Autodesk Inventor part; units mm, degrees
ref_plane "YZ Plane" through (0, 0, 0) normal (1, 0, 0) x (0, 1, 0)
ref_plane "XZ Plane" through (0, 0, 0) normal (0, 1, 0) x (-1, 0, 0)
ref_plane "XY Plane" through (0, 0, 0) normal (0, 0, 1) x (1, 0, 0)
sketch "Sketch1" plane through (0, 0, 0) normal (0, 1, 0) x (-1, 0, 0)
  circle A0 centre (0, 0) radius 12.7
  dimension "d0" = 25.4
extrude "Extrusion1" add sketch "Sketch1" along normal blind 25.4
sketch "Sketch2" plane through (0, 25.4, 0) normal (0, 1, 0) x (1, 0, 0)
  circle A0 centre (0, 0) radius 15.875
  dimension "d3" = 31.75
extrude "Extrusion2" add sketch "Sketch2" along normal blind 5.08
sketch "Sketch3" plane through (0, 0, 0) normal (0, -1, 0) x (1, 0, 0)
  circle A0 centre (0, 0) radius 12.7
extrude "Extrusion3" add sketch "Sketch3" along normal blind 6.35
chamfer "Chamfer1" distance 3.175 distance2 6.35 1 edges at (-12.7, -6.35, 0) measured on face at (0.3934, -6.35, -3.2397)
sketch "Sketch4" plane through (0, 30.48, 0) normal (0, 1, 0) x (1, 0, 0)
  line L0 (0, 0) -> (1.016, 0) construction
  line L1 (0, 0) -> (-1.016, 0) construction
  line L2 (-1.016, 0) -> (-3.556, 0) construction
  line L3 (-3.556, 0) -> (-3.556, 6.35) construction
  line L4 (-3.556, 6.35) -> (-1.016, 6.35) construction
  line L5 (-1.016, 6.35) -> (-1.016, 0) construction
  line L6 (-1.016, 6.35) -> (-6.096, 6.35)
  line L7 (-6.096, 6.35) -> (-6.096, -6.35)
  line L8 (-6.096, -6.35) -> (-1.016, -6.35)
  line L9 (-1.016, -6.35) -> (-1.016, 6.35)
  line L10 (1.016, 0) -> (1.016, 7.239) construction
  line L11 (1.016, 0) -> (6.096, 0) construction
  line L12 (3.556, 0) -> (3.556, 4.572) construction
  line L13 (3.556, 0) -> (3.556, -4.572) construction
  line L14 (3.556, 4.572) -> (4.826, 4.572) construction
  line L15 (3.556, -4.572) -> (2.286, -4.572) construction
  line L16 (4.826, 4.572) -> (3.556, 4.572)
  line L17 (3.556, 4.572) -> (3.556, -4.572)
  line L18 (3.556, -4.572) -> (4.826, -4.572)
  line L19 (4.826, -4.572) -> (4.826, 4.572)
  line L20 (1.016, 7.239) -> (6.096, 7.239) construction
  line L21 (6.096, 7.239) -> (3.5838, 7.239)
  line L22 (1.016, 4.6712) -> (1.016, -4.6712)
  line L23 (3.5838, -7.239) -> (6.096, -7.239)
  line L24 (6.096, -7.239) -> (6.096, 7.239)
  line L25 (-2.286, 0) -> (-3.556, 0)
  line L26 (-3.556, 0) -> (-3.556, 5.08)
  line L27 (-3.556, 5.08) -> (-2.286, 5.08)
  line L28 (-2.286, 5.08) -> (-2.286, 0)
  line L29 (-2.286, 0) -> (-3.556, 0)
  line L30 (-3.556, 0) -> (-3.556, -5.08)
  line L31 (-3.556, -5.08) -> (-2.286, -5.08)
  line L32 (-2.286, -5.08) -> (-2.286, 0)
  line L33 (1.016, 7.239) -> (1.016, 5.334) construction
  line L34 (1.016, -7.239) -> (1.016, -5.334) construction
  line L35 (1.016, -7.239) -> (2.921, -7.239) construction
  line L36 (1.016, 7.239) -> (2.921, 7.239) construction
  line L37 (2.4523, 6.7703) -> (1.4847, 5.8027)
  line L38 (1.4847, -5.8027) -> (2.4523, -6.7703)
  arc A0 (3.5838, 7.239) -> (2.4523, 6.7703) centre (3.5838, 5.6388) ccw
  arc A1 (1.4847, 5.8027) -> (1.016, 4.6712) centre (2.6162, 4.6712) ccw
  arc A2 (1.016, -4.6712) -> (1.4847, -5.8027) centre (2.6162, -4.6712) ccw
  arc A3 (2.4523, -6.7703) -> (3.5838, -7.239) centre (3.5838, -5.6388) ccw
  dimension "d11" = 1.016
  dimension "d12" = 1.016
  dimension "d13" = 2.54
  dimension "d14" = 6.35
  dimension "d15" = 5.08
  dimension "d16" = 12.7
  dimension "d17" = 7.239
  dimension "d18" = 5.08
  dimension "d19" = 4.572
  dimension "d20" = 4.572
  dimension "d21" = 1.27
  dimension "d22" = 1.27
  dimension "d23" = 5.08
  dimension "d24" = 14.478
  dimension "d25" = 5.08
  dimension "d26" = 5.08
  dimension "d27" = 1.905
  dimension "d28" = 1.905
  dimension "d29" = 1.905
  dimension "d30" = 1.905
  dimension "d31" = 1.6002
extrude "Extrusion4" cut sketch "Sketch4" against normal blind 6.35
properties part number "usbHdmiPanelMount" material "ABS Plastic"
The model under review builds one solid part; all positions refer to its coordinate system, in mm. A direction names the side the tool comes from. Round coordinates to 2 decimals unless told otherwise and drop trailing zeros. Loops run counter-clockwise (first coordinate to the right, second up) from the corner with the lowest first, then second, coordinate; pieces in that order, holes last. Notation, with made-up numbers: (27.25, 37.5) -> (73.25, 37.5) arc R20 cw to (73.25, 64.5) -> close; hole circle Ø8 at (-30.75, -35). An arc over 180 degrees is marked (long way). Answer as a JSON object with one key per item and string values. Group by question number.
1) Mouldability with a two-part tool opening along X and no side actions: class faces 1 (the face through (0, 30.48, 0)), 2 (the face through (3, 24.13, 0)), 3 (the face through (-1.016, 27, 0)) as released by +X, released by -X, zero draft, split by the parting line, or undercut.
2) We need section C-C on y = 15.5. Write out the cut boundary in (x, z), then the cut area to 3 significant figures.
3) For pin 1 Ø1.5 at (y, z) = (11, -12.5) entering from +X; pin 2 Ø5.5 at (x, y) = (-3, 28) entering from +Z; pin 3 Ø0.6 at (x, y) = (4, 27) entering from +Z, all flat-tipped, find the tip position at first contact; note any pin that passes through.
4) For line 1 (X direction, y = 25, z = -3.5); line 2 (X direction, y = 26, z = -3); line 3 (X direction, y = 0.5, z = 11), list the stretches that pass through material, from the lowest coordinate up. Write a range as [from, to].
5) For faces 4 (the face through (4, 30.48, 0)), 5 (the face through (-2.286, 27, 0)), list the 3-axis set-ups (+Z, -Z, +X, -X, +Y, -Y) from which the entire face can be reached by the end or side of a thin tool; tool diameter is ignored.
Result set:
{
 "1": {"face 1": "zero draft", "face 2": "undercut", "face 3": "undercut"},
 "2": {"outline": "circle Ø25.4 at (0, 0)", "area": "507 mm²"},
 "3": {"pin 1": "x = 4.82", "pin 2": "z = 15.87", "pin 3": "z = 15.44"},
 "4": {"line 1": "[-12.21, -6.1], [-3.56, -2.29], [-1.02, 1.02], [3.56, 4.83], [6.1, 12.21]", "line 2": "[-15.59, -6.1], [-3.56, -2.29], [-1.02, 1.02], [3.56, 4.83], [6.1, 15.59]", "line 3": "[-6.35, 6.35]"},
 "5": {"face 4": "+Z, -Z, +X, -X, +Y", "face 5": "+Y"}
}
